Part print with two shaded views. Sizes in mm from the minimum x, y, z corner. A direction names the side the tool comes from. Round coordinates to 2 decimals unless told otherwise and drop trailing zeros. Order: outer loops, then holes, each group sorted by start corner. A loop starts at its lowest first (then second) coordinate and runs counter-clockwise, first axis right, second up. Notation, with made-up numbers: (-10, 40) - (48, 40) arc R20 ccw to (48, 55) - close; hole circle Ø7 at (-9, 8). An arc over 180 degrees is marked (long way). Use one line per item in the form item = value.
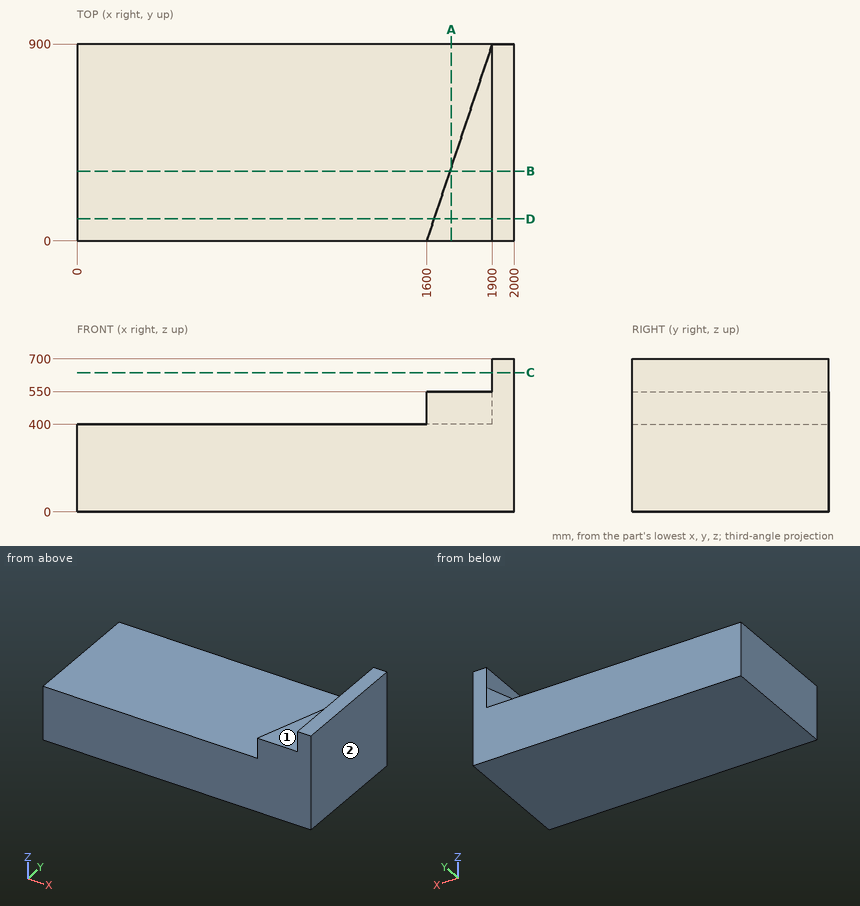
(1) Tool access for the marked faces 1 and 2: list every direction of +Z, -Z, +X, -X, +Y, -Y with a clear straight run to the whole face (end or side of a thin tool).
Report:
face_1 = +Z, -X, +Y, -Y
face_2 = +Z, -Z, +X, +Y, -Y
(2) Pin check, flat tips, straight feed: pin 1 (1.5 mm diameter, centred on x = 596.5, y = 531, fed in from +Z); pin 2 (6 mm diameter, centred on y = 216.5, z = 287.5, fed in from -X). Stop position of each tip, or through.
Report:
pin_1 = 400
pin_2 = 0
(3) Slice it at A-A on x = 1713. Give the cut face in (y, z), then the cut area to 3 significant figures.
Report:
outline = (0, 0) - (900, 0) - (900, 400) - (339, 400) - (339, 550) - (0, 550) - close
area = 411,000 mm2
(4) Slice it at C-C on z = 637. Give the cut face in (x, y).
Report:
outline = (1900, 0) - (2000, 0) - (2000, 900) - (1900, 900) - close
(5) Probe probe 1 along Z at (x, y) = (320, 101); probe 2 along X at (y, z) = (765.5, 585); probe 3 along X at (y, z) = (475.5, 427.5). List the from-to ranges inside material, lowest first. Write a range as [from, to].
Report:
probe_1 = [0, 400]
probe_2 = [1900, 2000]
probe_3 = [1758.5, 2000]
(6) Slice it at B-B on y = 318. Give the cut face in (x, z), then the cut area to 3 significant figures.
Report:
outline = (0, 0) - (2000, 0) - (2000, 700) - (1900, 700) - (1900, 550) - (1706, 550) - (1706, 400) - (0, 400) - close
area = 859,000 mm2
(7) Slice it at D-D on y = 100. Give the cut face in (x, z).
Report:
outline = (0, 0) - (2000, 0) - (2000, 700) - (1900, 700) - (1900, 550) - (1633.33, 550) - (1633.33, 400) - (0, 400) - close
